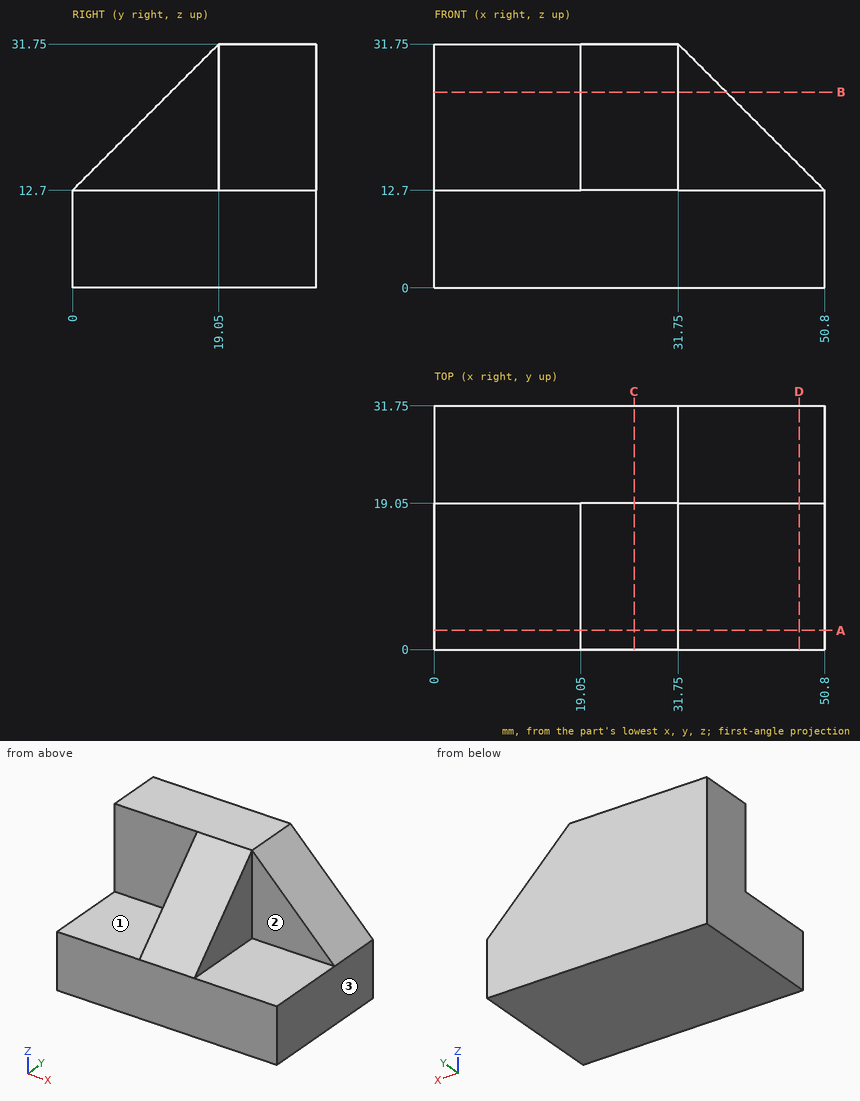
Can you work these out from the drawing? Everything is in mm from the part's minimum corner. A direction names the side the tool comes from. Round coordinates to 2 decimals unless told otherwise and drop trailing zeros. Write each loop counter-clockwise with the first axis right and the second up, starting at its lowest first coordinate (ties: lowest second). Pieces come first, ordered by that corner, then holes. Notation, with made-up numbers: (57, 48.5) - (66, 48.5) arc R29 ccw to (66, 76.5) - close; hole circle Ø2 at (46, 30). An arc over 180 degrees is marked (long way). Put each result on its own line as item: value. Start each with the question number.
(1) I want a section at D-D, the plane x = 47.5. Please give me the cut outline in (y, z).
(2) I want a section at A-A, the plane y = 2.5. Please give me the cut outline in (x, z).
(3) I want a section at B-B, the plane z = 25.5. Please give me the cut outline in (x, y), plus the area to 3 significant figures.
(4) I want a section at C-C, the plane x = 26. Please give me the cut outline in (y, z), plus the area to 3 significant figures.
(5) I need wall thicknesses on probe 1 along Y at (x, z) = (11, 21); probe 2 along Z at (x, y) = (39, 5). Which ranges of each line are inside material? Lowest first, please.
(6) Will these pins go through, and if not, where does the flat tip stop? pin 1 (5.5 mm diameter, centred on x = 13.5, z = 22.5, fed in from -Y); pin 2 (12 mm diameter, centred on y = 5.5, z = 21.5, fed in from -X); pin 3 (9.5 mm diameter, centred on x = 5.5, y = 6.5, fed in from +Z).
(7) For the marked faces 1, 2 and 3, which set-ups out of +Z, -Z, +X, -X, +Y, -Y let a thin tool reach every point of the face, with its end or its side?
Here are the results:
1. outline: (0, 0) - (31.75, 0) - (31.75, 16) - (19.05, 16) - (19.05, 12.7) - (0, 12.7) - close
2. outline: (0, 0) - (50.8, 0) - (50.8, 12.7) - (31.75, 12.7) - (31.75, 15.2) - (19.05, 15.2) - (19.05, 12.7) - (0, 12.7) - close
3. outline: (0, 19.05) - (19.05, 19.05) - (19.05, 12.8) - (31.75, 12.8) - (31.75, 19.05) - (38, 19.05) - (38, 31.75) - (0, 31.75) - close
3. area: 562 mm^2
4. outline: (0, 0) - (31.75, 0) - (31.75, 31.75) - (19.05, 31.75) - (0, 12.7) - close
4. area: 827 mm^2
5. probe 1: y = 19.05 to 31.75
5. probe 2: z = 0 to 12.7
6. pin 1: stops at y = 19.05
6. pin 2: stops at x = 19.05
6. pin 3: stops at z = 12.7
7. face 1: +Z, -X, -Y
7. face 2: +Z, +X, -Y
7. face 3: +Z, -Z, +X, +Y, -Y
